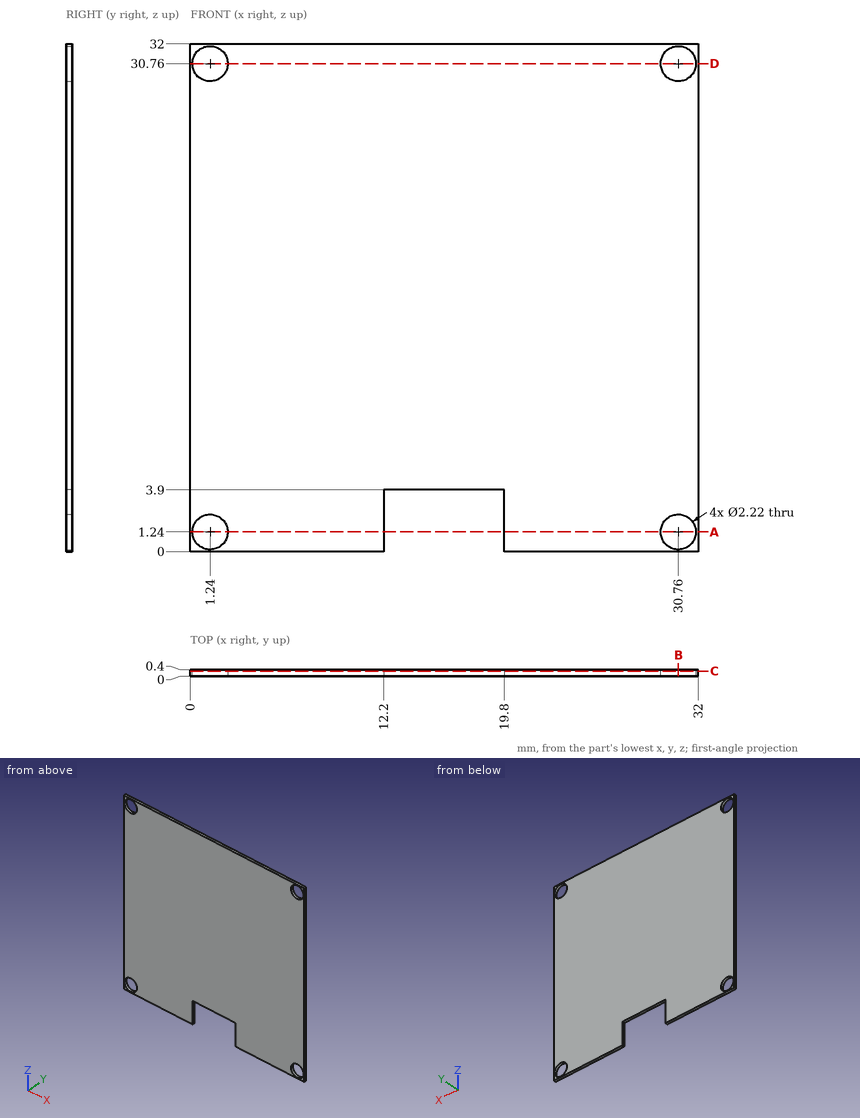
Print and shaded views of the part. All mm, measured from the part's lowest x, y and z. Coordinates: 2 decimals unless noted, no trailing zeros. Order: outer loops, then holes, each group sorted by start corner. A loop starts at its lowest first (then second) coordinate and runs counter-clockwise, first axis right, second up.
Item 1: Saw through at D-D on z = 30.76. List the corners of the cut face in (x, y).
Filled in:
outline: (0, 0) - (0.13, 0) - (0.13, 0.4) - (0, 0.4) - close; (2.35, 0) - (29.65, 0) - (29.65, 0.4) - (2.35, 0.4) - close; (31.87, 0) - (32, 0) - (32, 0.4) - (31.87, 0.4) - close
Item 2: Saw through at B-B on x = 30.76. List the corners of the cut face in (y, z), then the cut area to 3 significant figures.
Filled in:
outline: (0, 0) - (0.4, 0) - (0.4, 0.13) - (0, 0.13) - close; (0, 2.35) - (0.4, 2.35) - (0.4, 29.65) - (0, 29.65) - close; (0, 31.87) - (0.4, 31.87) - (0.4, 32) - (0, 32) - close
area: 11.0 mm2
Item 3: Saw through at A-A on z = 1.24. List the corners of the cut face in (x, y).
Filled in:
outline: (0, 0) - (0.13, 0) - (0.13, 0.4) - (0, 0.4) - close; (2.35, 0) - (12.2, 0) - (12.2, 0.4) - (2.35, 0.4) - close; (19.8, 0) - (29.65, 0) - (29.65, 0.4) - (19.8, 0.4) - close; (31.87, 0) - (32, 0) - (32, 0.4) - (31.87, 0.4) - close
Item 4: Saw through at C-C on y = 0.3. List the corners of the cut face in (x, z), then the cut area to 3 significant figures.
Filled in:
outline: (0, 0) - (12.2, 0) - (12.2, 3.9) - (19.8, 3.9) - (19.8, 0) - (32, 0) - (32, 32) - (0, 32) - close; hole circle Ø2.22 at (1.24, 1.24); hole circle Ø2.22 at (1.24, 30.76); hole circle Ø2.22 at (30.76, 1.24); hole circle Ø2.22 at (30.76, 30.76)
area: 979 mm2
Item 5: Drop a flat-ended pin along its axis: pin 1 Ø1.3 at (x, z) = (1.24, 30.76) entering from +Y. Give the stop position or say it passes through.
Filled in:
pin 1: passes through
Item 6: Drill centre lines: L1, parallel to X at y = 0.2, z = 30.5; L2, parallel to Z at x = 19, y = 0.2. Where is each one in solid material? Low to high.
Filled in:
L1: x = 0 to 0.16, 2.32 to 29.68, 31.84 to 32
L2: z = 3.9 to 32
